The drawing under review shows one solid part. Ordinate dimensions are in mm from its lowest x, y, z. Round coordinates to 2 decimals unless told otherwise and drop trailing zeros. Order: outer loops, then holes, each group sorted by start corner. A loop starts at its lowest first (then second) coordinate and runs counter-clockwise, first axis right, second up.
1) Mouldability with a two-part tool opening along X and no side actions: class the marked faces 1, 2 and 3 as pulls with the +X half, pulls with the -X half, needs draft (parallel to the pull), parting line crosses it, or undercut.
2) Consider section A-A (y = 7). Give the boundary of the cut face in (x, z), then the cut area to 3 significant figures.
3) Consider section C-C (z = 122). Give the boundary of the cut face in (x, y), then the cut area to 3 significant figures.
4) To check wall thickness, follow L1, parallel to X at y = 57.5, z = 89; L2, parallel to X at y = 23.5, z = 135; L3, parallel to X at y = 22, z = 89. State the ranges of each line that lie inside material, in increasing order.
5) Consider section B-B (y = 42.5). Give the boundary of the cut face in (x, z).
6) Consider section D-D (x = 85). Give the boundary of the cut face in (y, z).
7) Clearance check with flat-ended pins moving along their axes: P1, Ø4, axis at x = 124, y = 45, coming from the -Z side; P2, Ø10, axis at x = 63.5, y = 20.5, coming from the +Z side; P3, Ø6, axis at x = 98.5, y = 54, coming from the -Z side. State where each tip first meets the part, or that it passes through.
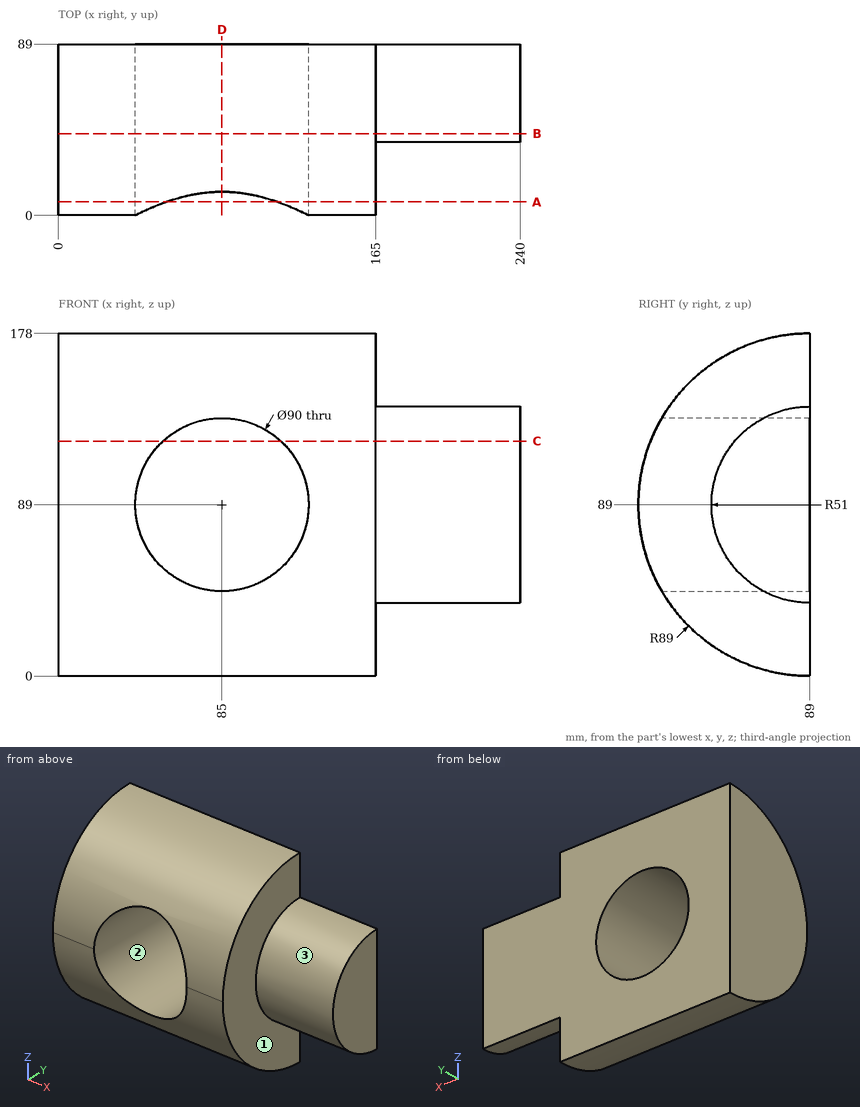
Answer below:
1. face 1: pulls with the +X half
1. face 2: undercut
1. face 3: needs draft
2. outline: (0, 54.4) - (56.23, 54.4) arc R45 cw to (56.23, 123.6) - (0, 123.6) - close; (113.77, 54.4) - (165, 54.4) - (165, 123.6) - (113.77, 123.6) arc R45 cw to start
2. area: 5,870 mm2
3. outline: (0, 6.34) - (54.41, 6.34) - (54.41, 89) - (0, 89) - close; (115.59, 6.34) - (165, 6.34) - (165, 50.12) - (240, 50.12) - (240, 89) - (115.59, 89) - close
3. area: 11,500 mm2
4. L1: x = 0 to 40, 130 to 240
4. L2: x = 0 to 165
4. L3: x = 0 to 40, 130 to 165
5. outline: (0, 13.11) - (165, 13.11) - (165, 68.05) - (240, 68.05) - (240, 109.95) - (165, 109.95) - (165, 164.89) - (0, 164.89) - close; hole circle Ø90 at (85, 89)
6. outline: (12.21, 44) arc R89 ccw to (89, 0) - (89, 44) - close; (12.21, 134) - (89, 134) - (89, 178) arc R89 ccw to start
7. P1: stops at z = 10.53
7. P2: stops at z = 151.36
7. P3: stops at z = 5.95
